Work out the finished part from the listing and answer in its coordinate system (mm). Round coordinates to 2 decimals unless told otherwise and drop trailing zeros. Loops run counter-clockwise (first coordinate to the right, second up) from the corner with the lowest first, then second, coordinate; pieces in that order, holes last. Notation, with made-up numbers: (-30.5, 10.5) - (-8.5, 10.5) arc R18 cw to (-8.5, 27.5) - close; hole circle Ø11 at (76.5, -27.5). An arc over 180 degrees is marked (long way). Return JSON: item names as keys, results as strings.
from build123d import *

# Parameters (mm, degrees)
SKETCH1_R           = 1.6
SKETCH1_R_2         = 30.5
SKETCH1_R_3         = 1.5
BOSS_EXTRUDE1_DEPTH = 2


with BuildPart() as part:
    # Sketch1 → Boss-Extrude1 (new body)
    with BuildSketch(Plane(origin=(0, 0, 0), x_dir=(1, 0, 0), z_dir=(0, 1, 0))):
        with BuildLine():
            Line((17.897079586, 48.929734976), (40.149284407, 43.651218265))
            ThreePointArc((40.149284407, 43.651218265), (42.540265174, 42.312242187), (43.866371506, 39.91409958))
            Line((43.866371506, 39.91409958), (49.02521675, 17.633846579))
            ThreePointArc((49.02521675, 17.633846579), (49.23478351, 16.809026698), (49.479249782, 15.993868858))
            ThreePointArc((49.479249782, 15.993868858), (51.999812242, -0.139738387), (49.392575566, -16.259565766))
            ThreePointArc((49.392575566, -16.259565766), (49.143731732, -17.073397941), (48.929734976, -17.897079586))
            Line((48.929734976, -17.897079586), (43.651218265, -40.149284407))
            ThreePointArc((43.651218265, -40.149284407), (42.312242187, -42.540265174), (39.91409958, -43.866371506))
            Line((39.91409958, -43.866371506), (17.633846579, -49.02521675))
            ThreePointArc((17.633846579, -49.02521675), (16.809026698, -49.23478351), (15.993868858, -49.479249782))
            ThreePointArc((15.993868858, -49.479249782), (-0.139738387, -51.999812242), (-16.259565766, -49.392575566))
            ThreePointArc((-16.259565766, -49.392575566), (-17.073397941, -49.143731732), (-17.897079586, -48.929734976))
            Line((-17.897079586, -48.929734976), (-40.149284407, -43.651218265))
            ThreePointArc((-40.149284407, -43.651218265), (-42.540265174, -42.312242187), (-43.866371506, -39.91409958))
            Line((-43.866371506, -39.91409958), (-49.02521675, -17.633846579))
            ThreePointArc((-49.02521675, -17.633846579), (-49.23478351, -16.809026698), (-49.479249782, -15.993868858))
            ThreePointArc((-49.479249782, -15.993868858), (-51.999812242, 0.139738387), (-49.392575566, 16.259565766))
            ThreePointArc((-49.392575566, 16.259565766), (-49.143731732, 17.073397941), (-48.929734976, 17.897079586))
            Line((-48.929734976, 17.897079586), (-43.651218265, 40.149284407))
            ThreePointArc((-43.651218265, 40.149284407), (-42.312242187, 42.540265174), (-39.91409958, 43.866371506))
            Line((-39.91409958, 43.866371506), (-17.633846579, 49.02521675))
            ThreePointArc((-17.633846579, 49.02521675), (-16.809026698, 49.23478351), (-15.993868858, 49.479249782))
            ThreePointArc((-15.993868858, 49.479249782), (-8.026622704, 51.3767781), (0.139738387, 51.999812242))
            ThreePointArc((0.139738387, 51.999812242), (8.302633013, 51.332896714), (16.259565766, 49.392575566))
            ThreePointArc((16.259565766, 49.392575566), (17.073397941, 49.143731732), (17.897079586, 48.929734976))
        make_face()
        with Locations(Location((-38.8907, 38.8907, 0), (0, 0, 270))):
            Circle(SKETCH1_R, mode=Mode.SUBTRACT)
        with Locations(Location((38.8907, 38.8907, 0), (0, 0, 90))):
            Circle(SKETCH1_R, mode=Mode.SUBTRACT)
        with Locations(Location((38.8907, -38.8907, 0), (0, 0, 270))):
            Circle(SKETCH1_R, mode=Mode.SUBTRACT)
        with Locations(Location((-38.8907, -38.8907, 0), (0, 0, 90))):
            Circle(SKETCH1_R, mode=Mode.SUBTRACT)
        with Locations(Location((0, 0, 0), (0, 0, 270))):
            Circle(SKETCH1_R_2, mode=Mode.SUBTRACT)
        with Locations(Location((0, 34.1739971, 0), (0, 0, 270))):
            Circle(SKETCH1_R_3, mode=Mode.SUBTRACT)
        with Locations(Location((-29.672696408, -17.456745562, 0), (0, 0, 270))):
            Circle(SKETCH1_R_3, mode=Mode.SUBTRACT)
        with Locations(Location((29.672696408, -16.717251537, 0), (0, 0, 270))):
            Circle(SKETCH1_R_3, mode=Mode.SUBTRACT)
    extrude(amount=BOSS_EXTRUDE1_DEPTH)


solid = part.part
1) Find the intervals of material crossed by L1, parallel to X at y = 1, z = 16.5; L2, parallel to X at y = 0.6, z = -39; L3, parallel to X at y = 1.35, z = 0, in increasing order.
Verdict:
{"L1": "x = -49.32 to -30.83, -28.52 to -25.65, 25.65 to 28.19, 31.16 to 49.32", "L2": "x = -43.92 to -40.49, -37.29 to 37.29, 40.49 to 44.08", "L3": "x = -52 to -30.5, 30.5 to 52"}
2) A flat-ended cylindrical pin translates along its axis: pin 1 (4 mm diameter, centred on x = 38.89, z = 38.89, fed in from -Y). Find the tip coordinate at first contact, or state that the pin passes through.
Verdict:
{"pin 1": "stops at y = 0"}
3) Determine the mould class of faces 1 (the cylindrical face through (-39.864, 0.986, -40.16)), 2 (the flat face through (28.867, 0.986, -46.327)), 3 (the cylindrical face through (-42.51, 0.99, 42.34)) for opening direction Z: pulls with the +Z half, pulls with the -Z half, needs draft (parallel to the pull), parting line crosses it, or undercut.
Verdict:
{"face 1": "undercut", "face 2": "pulls with the -Z half", "face 3": "pulls with the +Z half"}
4) Section C-C (x = -20) is taken. Give the vertices of the cut face in (y, z).
Verdict:
{"outline": "(0, -48.48) - (2, -48.48) - (2, -23.03) - (0, -23.03) - close; (0, 23.03) - (2, 23.03) - (2, 48.43) - (0, 48.43) - close"}
5) Section A-A (z = 0) is taken. Give the vertices of the cut face in (x, y), and give its area (3 significant figures).
Verdict:
{"outline": "(-52, 0) - (-30.5, 0) - (-30.5, 2) - (-52, 2) - close; (30.5, 0) - (52, 0) - (52, 2) - (30.5, 2) - close", "area": "86.0 mm2"}
6) Section B-B (y = 1.65) is taken. Count the separate pieces of the cut face and the enclosed holes in it, and give its area (3 significant figures).
Verdict:
{"separate pieces": "1", "enclosed holes": "8", "area": "6,160 mm2"}
7) Section D-D (z = 46) is taken. Give the vertices of the cut face in (x, y), and give its area (3 significant figures).
Verdict:
{"outline": "(-30.25, 0) - (30.7, 0) - (30.7, 2) - (-30.25, 2) - close", "area": "122 mm2"}
